Source: three-view drawing plus pictorial views. Frame: mm from the lowest corner of the part. Coordinates: 2 decimals unless noted, no trailing zeros. Loops run counter-clockwise (first coordinate to the right, second up) from the corner with the lowest first, then second, coordinate; pieces in that order, holes last. Notation, with made-up numbers: M 8.25,85.5 L 47.25,85.5 A7 cw 47.25,91.5 Z; hole C 83,-34 d10. An arc over 180 degrees is marked long. Use a Markdown table: item, result. Add a question column.
1. Line query: L1, parallel to Z at x = 38, y = 13; L2, parallel to Y at x = 15.5, z = 24.5; L3, parallel to X at y = 18.5, z = 6 (1 decimal). Output: solid intervals per line, ascending. Write a range as [from, to].
2. Section A-A on x = 20. Output: boundary loops of the cut face in (y, z).
3. Section C-C on z = 18. Output: boundary loops of the cut face in (x, y), then the cut area to 3 significant figures.
4. Section D-D on z = 11. Output: boundary loops of the cut face in (x, y).
5. Pin query (flat end, axial travel): pin 1 (2 mm diameter, centred on x = 10, z = 3.5, fed in from +Y) (1 decimal); pin 2 (1.5 mm diameter, centred on x = 26, z = 8.5, fed in from +Y); pin 3 (4 mm diameter, centred on x = 16, y = 30, fed in from +Z). Return the tip coordinate at first contact, or that it passes through.
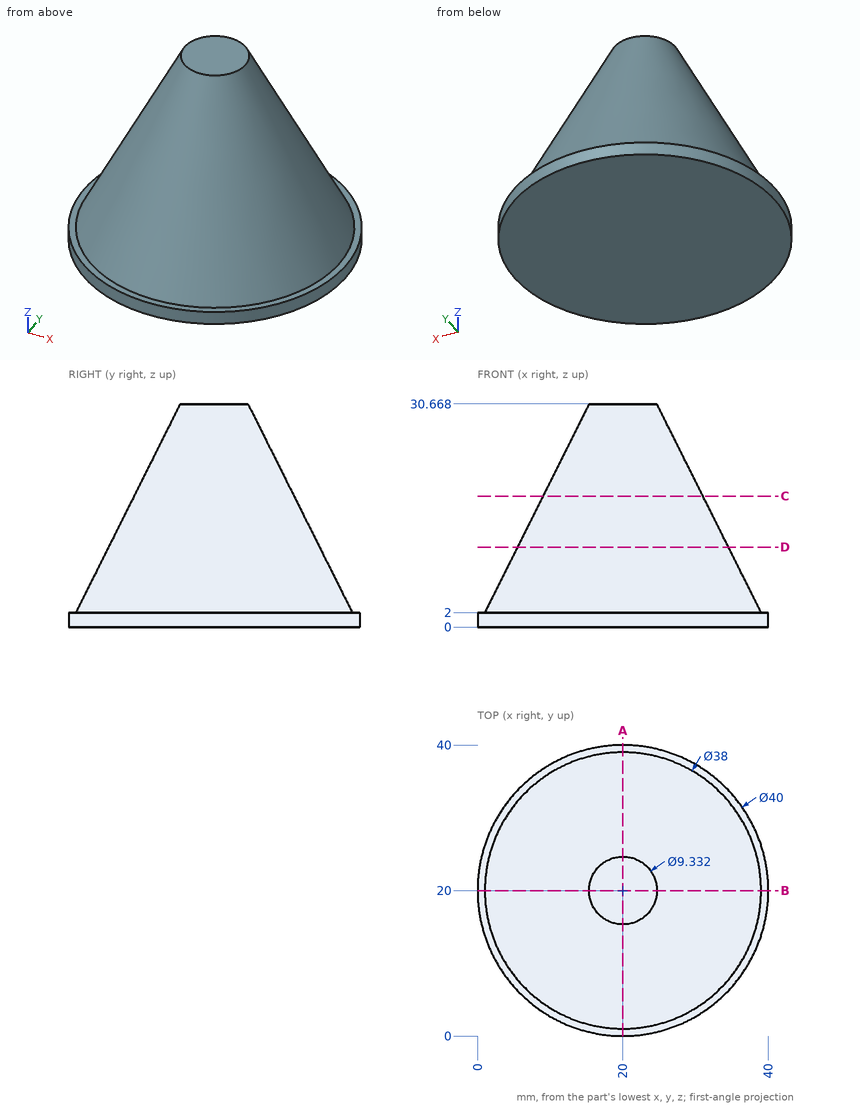
Answers below:
| question | item | result |
|---|---|---|
| 1 | L1 | z = [0, 2] |
| 1 | L2 | y = [13.69, 26.31] |
| 1 | L3 | x = [3.1, 36.9] |
| 2 | outline | M 0,0 L 40,0 L 40,2 L 39,2 L 24.67,30.67 L 15.33,30.67 L 1,2 L 0,2 Z |
| 3 | outline | C 20,20 d22 |
| 3 | area | 380 mm² |
| 4 | outline | C 20,20 d29 |
| 5 | pin 1 | stops at y = 36.1 |
| 5 | pin 2 | stops at y = 35.06 |
| 5 | pin 3 | stops at z = 22.46 |
